Build history of the part. All positions in model axes, mm. A direction names the side the tool comes from. Round coordinates to 2 decimals unless told otherwise and drop trailing zeros. Loops run counter-clockwise (first coordinate to the right, second up) from the corner with the lowest first, then second, coordinate; pieces in that order, holes last. Notation, with made-up numbers: (-14.5, 35.5) - (5.5, 35.5) arc R30 ccw to (5.5, 66.5) - close; hole circle Ø7 at (73.25, -13). An arc over 180 degrees is marked (long way). Use one line per item in the form item = value. Start each with the question number.
Q1. Drill centre lines: line 1 (Z direction, x = 0, y = -0.1) (3 decimals); line 2 (X direction, y = -2.4, z = -2); line 3 (X direction, y = 0.6, z = 1.25). Where is each one in solid material? Low to high.
Q2. Pin check, flat tips, straight feed: pin 1 (1 mm diameter, centred on x = 3.5, y = -2.5, fed in from -Z); pin 2 (1 mm diameter, centred on y = -2, z = -3, fed in from +X); pin 3 (0.6 mm diameter, centred on y = 0.5, z = -2.5, fed in from +X); pin 4 (0.8 mm diameter, centred on x = -4, z = 1, fed in from +Y). Stop position of each tip, or through.
Q3. Mould opens along Z. For faces 4 (the face through (0, -2, 5)), 5 (the face through (0, -3.6, -4)), 6 (the face through (2.88, -1.32, -0.93)) say: released by +Z, released by -Z, zero draft, split by the parting line, or undercut.
Q4. Saw through at A-A (x = 0). Give the cut face in (y, z) (3 decimals).
Q5. 3-axis set-ups, long thin cutter, end or side, ignore diameter. For faces 1 (the face through (0, -3.6, 4)), 2 (the face through (-4, 0, 0)), 3 (the face through (4, 0, 0)): which of +Z, -Z, +X, -X, +Y, -Y reach the whole face in a straight line?
Q6. Saw through at C-C (z = 1.5). Give the cut face in (x, y).
Q7. Saw through at D-D (y = -3.05). Give the cut face in (x, z) (3 decimals).
Q8. Saw through at B-B (z = -3.5). Give the cut face in (x, y), then the cut area to 3 significant figures.
```python
from build123d import *

# Parameters (mm, degrees)
EXTRUDE_BODY_DEPTH = 10
SKETCH2_W          = 1.9
SKETCH2_H          = 0.9
CUT_EXTRUDE1_DEPTH = 12.703418304
SKETCH3_W          = 1.9
SKETCH3_H          = 0.9
CUT_EXTRUDE2_DEPTH = 12.703418304
CUT_EXTRUDE3_DEPTH = 12.703418304
HOLE_REVOLVE_D     = 6.05
EDGE_FILLETS_R     = 0.2


with BuildPart() as part:
    # Sketch1 → Extrude Body (new body)
    with BuildSketch(Plane.XY.offset(5)):
        Polygon((4.9, -1), (4.9, 0.9), (-4.9, 0.9), (-4.9, -1), (-2.3, -3.6), (2.3, -3.6), align=None)
    extrude(amount=-EXTRUDE_BODY_DEPTH)

    # Sketch2 → Cut-Extrude1 (cut, through all)
    with BuildSketch(Plane(origin=(0, 0, -5), x_dir=(-1, 0, 0), z_dir=(0, 0, -1))):
        with Locations((3.95, 0.45)):
            Rectangle(SKETCH2_W, SKETCH2_H)
    extrude(amount=-CUT_EXTRUDE1_DEPTH, mode=Mode.SUBTRACT)

    # Sketch3 → Cut-Extrude2 (cut, through all)
    with BuildSketch(Plane(origin=(0, 0, -5), x_dir=(-1, 0, 0), z_dir=(0, 0, -1))):
        with Locations((-3.95, 0.45)):
            Rectangle(SKETCH3_W, SKETCH3_H)
    extrude(amount=-CUT_EXTRUDE2_DEPTH, mode=Mode.SUBTRACT)

    # Sketch4 → Cut-Extrude3 (cut, through all)
    with BuildSketch(Plane(origin=(0, 0, -5), x_dir=(-1, 0, 0), z_dir=(0, 0, -1))):
        Polygon((0.4, 0.9), (-0.4, 0.9), (0, 0.5), align=None)
    extrude(amount=-CUT_EXTRUDE3_DEPTH, mode=Mode.SUBTRACT)

    # Hole Revolve (through all)
    with Locations(Plane(origin=(0, -3.6, 0), x_dir=(-1, 0, 0), z_dir=(0, -1, 0))):
        with Locations((0, 0)):
            Hole(HOLE_REVOLVE_D / 2)

    # Edge Fillets
    # the kernel refuses this fillet: 0.2 mm, written as the material it adds along each edge
    with BuildSketch(Plane(origin=(3, 0, -5), x_dir=(1, 0, 0), z_dir=(0, 0, 1))) as edge_fillets_piece_1_section:
        with BuildLine():
            CenterArc((EDGE_FILLETS_R, EDGE_FILLETS_R), EDGE_FILLETS_R, 180, 90)
            Line((0, EDGE_FILLETS_R), (0, 0))
            Line((0, 0), (EDGE_FILLETS_R, 0))
        make_face()
    edge_fillets_piece_1 = extrude(amount=5.111895633, mode=Mode.PRIVATE)
    edge_fillets_piece_1 = edge_fillets_piece_1 - Plane(origin=(0, 0.044194975, 0), x_dir=(1, 0, 0), z_dir=(0, 1, 0)) * Cylinder(3.025, 12, mode=Mode.PRIVATE)
    add(edge_fillets_piece_1)
    with BuildSketch(Plane(origin=(3, 0, -0.111895633), x_dir=(1, 0, 0), z_dir=(0, 0, 1))) as edge_fillets_piece_2_section:
        with BuildLine():
            CenterArc((EDGE_FILLETS_R, EDGE_FILLETS_R), EDGE_FILLETS_R, 180, 90)
            Line((0, EDGE_FILLETS_R), (0, 0))
            Line((0, 0), (EDGE_FILLETS_R, 0))
        make_face()
    edge_fillets_piece_2 = extrude(amount=5.111895633, mode=Mode.PRIVATE)
    edge_fillets_piece_2 = edge_fillets_piece_2 - Plane(origin=(0, 0.044194976, 0), x_dir=(1, 0, 0), z_dir=(0, 1, 0)) * Cylinder(3.025, 12, mode=Mode.PRIVATE)
    add(edge_fillets_piece_2)
    with BuildSketch(Plane(origin=(-3, 0, -0.111895633), x_dir=(-1, 0, 0), z_dir=(0, 0, 1))) as edge_fillets_piece_3_section:
        with BuildLine():
            CenterArc((EDGE_FILLETS_R, -EDGE_FILLETS_R), EDGE_FILLETS_R, 90, 90)
            Line((0, -EDGE_FILLETS_R), (0, 0))
            Line((0, 0), (EDGE_FILLETS_R, 0))
        make_face()
    edge_fillets_piece_3 = extrude(amount=5.111895633, mode=Mode.PRIVATE)
    edge_fillets_piece_3 = edge_fillets_piece_3 - Plane(origin=(0, 0.044194976, 0), x_dir=(1, 0, 0), z_dir=(0, 1, 0)) * Cylinder(3.025, 12, mode=Mode.PRIVATE)
    add(edge_fillets_piece_3)
    with BuildSketch(Plane(origin=(-3, 0, -5), x_dir=(-1, 0, 0), z_dir=(0, 0, 1))) as edge_fillets_piece_4_section:
        with BuildLine():
            CenterArc((EDGE_FILLETS_R, -EDGE_FILLETS_R), EDGE_FILLETS_R, 90, 90)
            Line((0, -EDGE_FILLETS_R), (0, 0))
            Line((0, 0), (EDGE_FILLETS_R, 0))
        make_face()
    edge_fillets_piece_4 = extrude(amount=5.111895633, mode=Mode.PRIVATE)
    edge_fillets_piece_4 = edge_fillets_piece_4 - Plane(origin=(0, 0.044194976, 0), x_dir=(1, 0, 0), z_dir=(0, 1, 0)) * Cylinder(3.025, 12, mode=Mode.PRIVATE)
    add(edge_fillets_piece_4)
    with BuildSketch(Plane(origin=(0, 0.5, 2.525), x_dir=(-0.7071067811865454, 0.7071067811865497, 0), z_dir=(0, 0, 1))) as edge_fillets_piece_5_section:
        with BuildLine():
            CenterArc((EDGE_FILLETS_R, -EDGE_FILLETS_R), EDGE_FILLETS_R, 90, 90)
            Line((0, -EDGE_FILLETS_R), (0, 0))
            Line((0, 0), (EDGE_FILLETS_R, 0))
        make_face()
    edge_fillets_piece_5 = extrude(amount=2.475, mode=Mode.PRIVATE)
    edge_fillets_piece_5 = edge_fillets_piece_5 - Plane(origin=(0, 0.564041319, 0), x_dir=(1, 0, 0), z_dir=(0, 1, 0)) * Cylinder(3.025, 6, mode=Mode.PRIVATE)
    add(edge_fillets_piece_5)
    with BuildSketch(Plane(origin=(0, 0.5, -5), x_dir=(-0.7071067811865455, 0.7071067811865496, 0), z_dir=(0, 0, 1))) as edge_fillets_piece_6_section:
        with BuildLine():
            CenterArc((EDGE_FILLETS_R, -EDGE_FILLETS_R), EDGE_FILLETS_R, 90, 90)
            Line((0, -EDGE_FILLETS_R), (0, 0))
            Line((0, 0), (EDGE_FILLETS_R, 0))
        make_face()
    edge_fillets_piece_6 = extrude(amount=2.475, mode=Mode.PRIVATE)
    edge_fillets_piece_6 = edge_fillets_piece_6 - Plane(origin=(0, 0.564041319, 0), x_dir=(1, 0, 0), z_dir=(0, 1, 0)) * Cylinder(3.025, 6, mode=Mode.PRIVATE)
    add(edge_fillets_piece_6)
    # the kernel refuses this fillet: 0.2 mm, written as the material it takes off along each edge
    with BuildSketch(Plane(origin=(4.9, 0, -5.5), x_dir=(0, -1, 0), z_dir=(0, 0, 1))) as edge_fillets_2_piece_1:
        with BuildLine():
            CenterArc((EDGE_FILLETS_R, -EDGE_FILLETS_R), EDGE_FILLETS_R, 90, 90)
            Line((0, -EDGE_FILLETS_R), (0, 0))
            Line((0, 0), (EDGE_FILLETS_R, 0))
        make_face()
    extrude(amount=11, mode=Mode.SUBTRACT)
    with BuildSketch(Plane(origin=(-4.9, -1, 5.207106781), x_dir=(0.7071067811865468, -0.7071067811865481, 0), z_dir=(0, 0, -1)), Plane(origin=(4.9, -1, 5.207106781), x_dir=(0, 1, 0), z_dir=(0, 0, -1))) as edge_fillets_2_piece_2:
        with BuildLine():
            CenterArc((EDGE_FILLETS_R * 0.414213562373, -EDGE_FILLETS_R), EDGE_FILLETS_R, 90, 45)
            Line((-EDGE_FILLETS_R * 0.292893218813, -EDGE_FILLETS_R * 0.292893218813), (0, 0))
            Line((0, 0), (EDGE_FILLETS_R * 0.414213562373, 0))
        make_face()
    extrude(amount=10.414213562, mode=Mode.SUBTRACT)
    with BuildSketch(Plane(origin=(3, 0.9, -0.111895633), x_dir=(-1, 0, 0), z_dir=(0, 0, 1)), Plane(origin=(-3, 0.9, -0.111895633), x_dir=(0, -1, 0), z_dir=(0, 0, 1))) as edge_fillets_2_piece_3:
        with BuildLine():
            CenterArc((EDGE_FILLETS_R, EDGE_FILLETS_R), EDGE_FILLETS_R, 180, 90)
            Line((0, EDGE_FILLETS_R), (0, 0))
            Line((0, 0), (EDGE_FILLETS_R, 0))
        make_face()
    extrude(amount=5.611895633, mode=Mode.SUBTRACT)
    with BuildSketch(Plane(origin=(0.4, 0.9, -5.207106781), x_dir=(1, 0, 0), z_dir=(0, 0, 1)), Plane(origin=(-0.4, 0.9, -5.207106781), x_dir=(0.7071067811865449, -0.7071067811865502, 0), z_dir=(0, 0, 1))) as edge_fillets_2_piece_4:
        with BuildLine():
            CenterArc((EDGE_FILLETS_R * 0.414213562373, -EDGE_FILLETS_R), EDGE_FILLETS_R, 90, 45)
            Line((-EDGE_FILLETS_R * 0.292893218813, -EDGE_FILLETS_R * 0.292893218813), (0, 0))
            Line((0, 0), (EDGE_FILLETS_R * 0.414213562373, 0))
        make_face()
    extrude(amount=2.415776469, mode=Mode.SUBTRACT)
    with BuildSketch(Plane(origin=(-0.4, 0.9, 2.791330312), x_dir=(-1, 0, 0), z_dir=(0, 0, 1)), Plane(origin=(0.4, 0.9, 2.791330312), x_dir=(-0.7071067811865465, -0.7071067811865485, 0), z_dir=(0, 0, 1))) as edge_fillets_2_piece_5:
        with BuildLine():
            CenterArc((EDGE_FILLETS_R * 0.414213562373, EDGE_FILLETS_R), EDGE_FILLETS_R, 225, 45)
            Line((-EDGE_FILLETS_R * 0.292893218813, EDGE_FILLETS_R * 0.292893218813), (0, 0))
            Line((0, 0), (EDGE_FILLETS_R * 0.414213562373, 0))
        make_face()
    extrude(amount=2.415776469, mode=Mode.SUBTRACT)
    with BuildSketch(Plane(origin=(-4.9, 0, -5.5), x_dir=(0, -1, 0), z_dir=(0, 0, 1))) as edge_fillets_2_piece_6:
        with BuildLine():
            CenterArc((EDGE_FILLETS_R, EDGE_FILLETS_R), EDGE_FILLETS_R, 180, 90)
            Line((0, EDGE_FILLETS_R), (0, 0))
            Line((0, 0), (EDGE_FILLETS_R, 0))
        make_face()
    extrude(amount=11, mode=Mode.SUBTRACT)
    with BuildSketch(Plane(origin=(-2.3, -3.6, -1.757740541), x_dir=(-0.7071067811865448, 0.7071067811865502, 0), z_dir=(0, 0, -1))) as edge_fillets_2_piece_7:
        with BuildLine():
            CenterArc((EDGE_FILLETS_R * 0.414213562373, EDGE_FILLETS_R), EDGE_FILLETS_R, 225, 45)
            Line((-EDGE_FILLETS_R * 0.292893218813, EDGE_FILLETS_R * 0.292893218813), (0, 0))
            Line((0, 0), (EDGE_FILLETS_R * 0.414213562373, 0))
        make_face()
    extrude(amount=3.44936624, mode=Mode.SUBTRACT)
    with BuildSketch(Plane(origin=(2.3, -3.6, -1.757740541), x_dir=(0.7071067811865476, 0.7071067811865476, 0), z_dir=(0, 0, -1))) as edge_fillets_2_piece_8:
        with BuildLine():
            CenterArc((EDGE_FILLETS_R * 0.414213562373, -EDGE_FILLETS_R), EDGE_FILLETS_R, 90, 45)
            Line((-EDGE_FILLETS_R * 0.292893218813, -EDGE_FILLETS_R * 0.292893218813), (0, 0))
            Line((0, 0), (EDGE_FILLETS_R * 0.414213562373, 0))
        make_face()
    extrude(amount=3.44936624, mode=Mode.SUBTRACT)


solid = part.part
```
Report:
q1.line_1 = -5 to -3.025, 3.025 to 5
q1.line_2 = -3.5 to -2.27, 2.27 to 3.5
q1.line_3 = -3 to -2.75, 2.75 to 3
q2.pin_1 = -5
q2.pin_2 = 4.4
q2.pin_3 = 3
q2.pin_4 = 0
q3.face_4 = released by +Z
q3.face_5 = zero draft
q3.face_6 = undercut
q4.outline = (-3.6, -5) - (0.583, -5) - (0.583, -3.025) - (-3.6, -3.025) - close; (-3.6, 3.025) - (0.583, 3.025) - (0.583, 5) - (-3.6, 5) - close
q5.face_1 = +Z, -Z, +X, -X, -Y
q5.face_2 = +Z, -Z, -X, +Y
q5.face_3 = +Z, -Z, +X, +Y
q6.outline = (-4.9, -0.92) arc R0.2 ccw to (-4.84, -1.06) - (-2.63, -3.27) - (-2.63, 0.9) - (-2.8, 0.9) arc R0.2 ccw to (-3, 0.7) - (-3, 0.2) arc R0.2 cw to (-3.2, 0) - (-4.7, 0) arc R0.2 ccw to (-4.9, -0.2) - close; (2.63, -3.27) - (4.84, -1.06) arc R0.2 ccw to (4.9, -0.92) - (4.9, -0.2) arc R0.2 ccw to (4.7, 0) - (3.2, 0) arc R0.2 cw to (3, 0.2) - (3, 0.7) arc R0.2 ccw to (2.8, 0.9) - (2.63, 0.9) - close
q7.outline = (-2.85, -5) - (2.85, -5) - (2.85, -1.014) arc R3.025 cw to (-2.85, -1.014) - close; (-2.85, 1.014) arc R3.025 cw to (2.85, 1.014) - (2.85, 5) - (-2.85, 5) - close
q8.outline = (-4.9, -0.92) arc R0.2 ccw to (-4.84, -1.06) - (-2.36, -3.54) arc R0.2 ccw to (-2.22, -3.6) - (2.22, -3.6) arc R0.2 ccw to (2.36, -3.54) - (4.84, -1.06) arc R0.2 ccw to (4.9, -0.92) - (4.9, -0.2) arc R0.2 ccw to (4.7, 0) - (3.2, 0) arc R0.2 cw to (3, 0.2) - (3, 0.9) - (0.48, 0.9) arc R0.2 ccw to (0.34, 0.84) - (0.14, 0.64) arc R0.2 cw to (-0.14, 0.64) - (-0.34, 0.84) arc R0.2 ccw to (-0.48, 0.9) - (-3, 0.9) - (-3, 0.2) arc R0.2 cw to (-3.2, 0) - (-4.7, 0) arc R0.2 ccw to (-4.9, -0.2) - close
q8.area = 33.8 mm²
